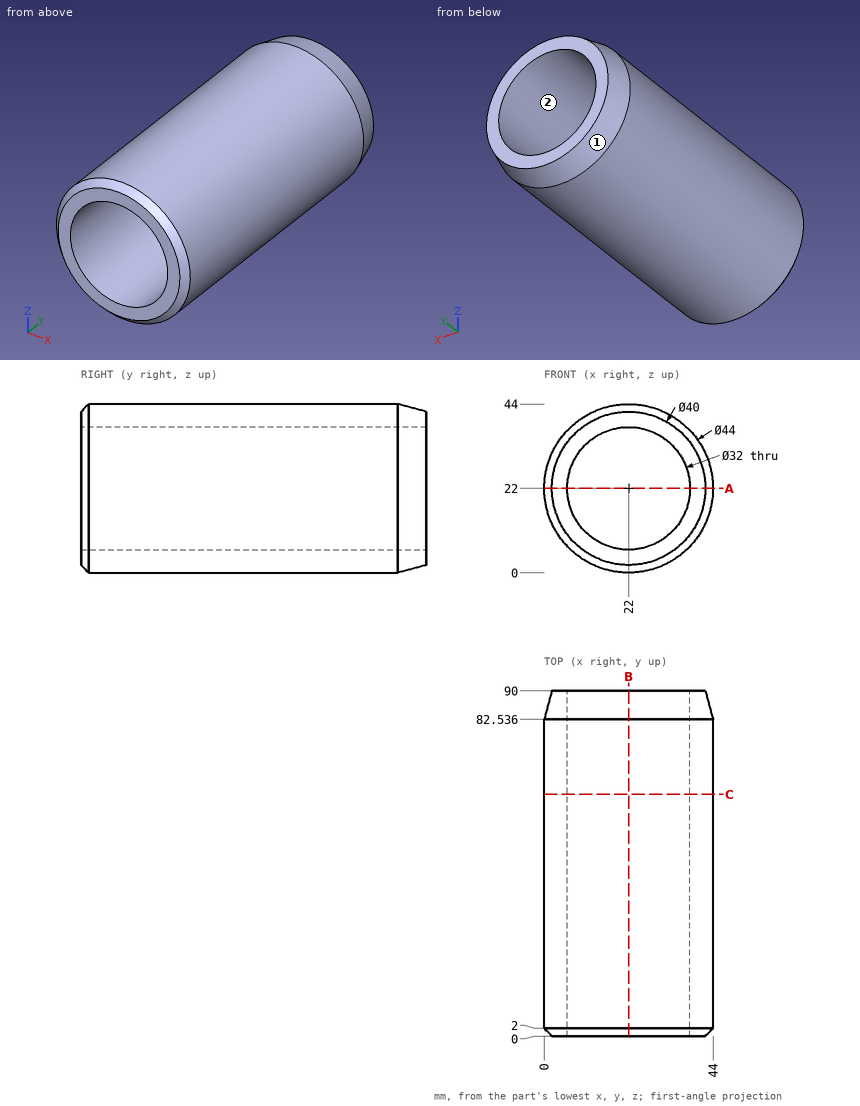
Answer from the drawing. Dimensions are ordinates in mm from the lowest x, y and z of the part. Round coordinates to 2 decimals unless told otherwise and drop trailing zeros. Order: outer loops, then holes, each group sorted by start corner. A loop starts at its lowest first (then second) coordinate and runs counter-clockwise, first axis right, second up.
1) Straight lines are drawn through the part: L1, parallel to X at y = 55, z = 22; L2, parallel to Z at x = 10, y = 68; L3, parallel to Z at x = 8, y = 82. For each, find the intervals that lie inside material, in ascending order.
2) The part is cut by section A-A on z = 22. Write down the section's boundary in (x, y).
3) The part is cut by section C-C on y = 63. Write down the section's boundary in (x, z), plus the area to 3 significant figures.
4) The mould has two halves that part along Z. Classify the marked faces 1 and 2: released by +Z, released by -Z, zero draft, split by the parting line, or undercut.
5) The part is cut by section B-B on x = 22. Write down the section's boundary in (y, z), plus the area to 3 significant figures.
6) Flat-ended cylindrical pins translate along their axes: pin 1 (12 mm diameter, centred on x = 29.5, y = 61, fed in from -Z); pin 2 (10 mm diameter, centred on x = 11.5, y = 17.5, fed in from +Z); pin 3 (3 mm diameter, centred on y = 59.5, z = 8, fed in from +X). Find the tip coordinate at first contact, or state that the pin passes through.
Resolved:
1. L1: x = 0 to 6, 38 to 44
1. L2: z = 3.56 to 11.42, 32.58 to 40.44
1. L3: z = 5.03 to 14.25, 29.75 to 38.97
2. outline: (0, 2) - (2, 0) - (6, 0) - (6, 90) - (2, 90) - (0, 82.54) - close; (38, 0) - (42, 0) - (44, 2) - (44, 82.54) - (42, 90) - (38, 90) - close
3. outline: circle Ø44 at (22, 22); hole circle Ø32 at (22, 22)
3. area: 716 mm2
4. face 1: split by the parting line
4. face 2: undercut
5. outline: (0, 2) - (2, 0) - (82.54, 0) - (90, 2) - (90, 6) - (0, 6) - close; (0, 38) - (90, 38) - (90, 42) - (82.54, 44) - (2, 44) - (0, 42) - close
5. area: 1,060 mm2
6. pin 1: stops at z = 0.05
6. pin 2: stops at z = 43.3
6. pin 3: stops at x = 40.1
